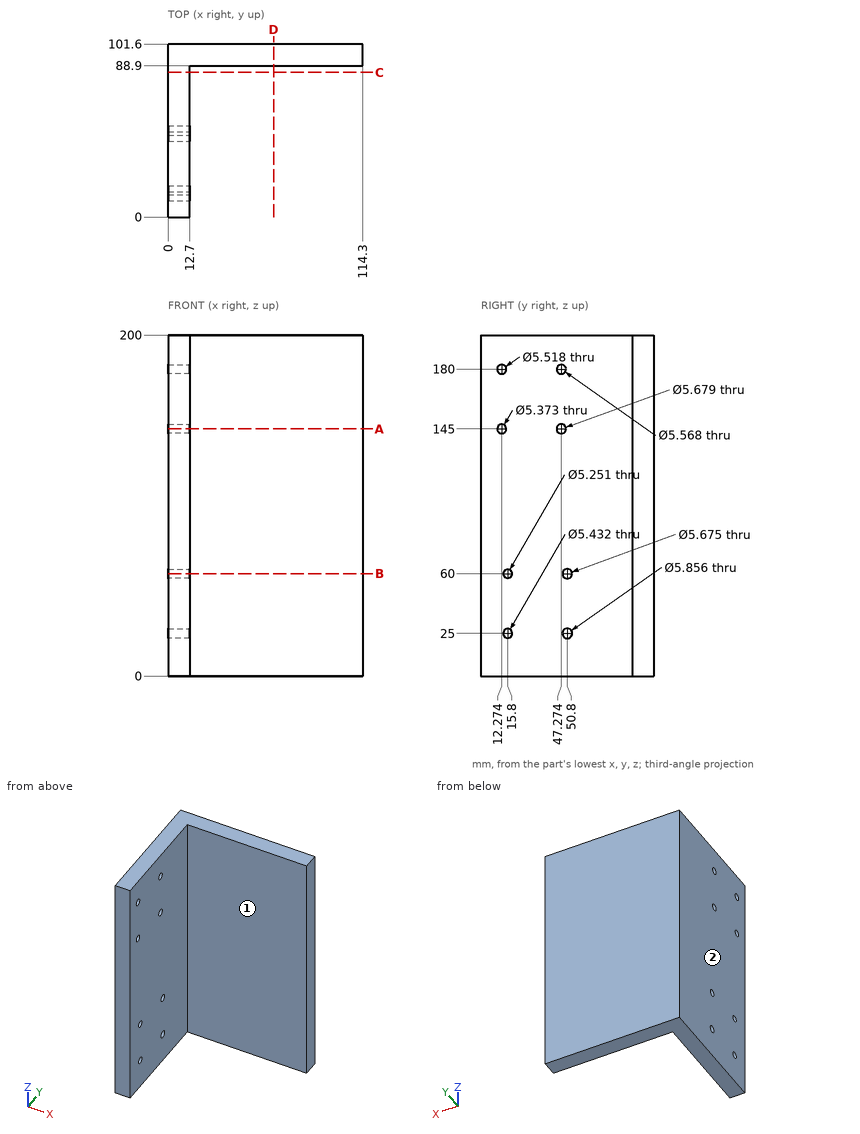
Could you check a few things on this drawing? It's one solid part, dimensions in mm from its lowest x, y, z. A direction names the side the tool comes from. Round coordinates to 2 decimals unless told otherwise and drop trailing zeros. Loops run counter-clockwise (first coordinate to the right, second up) from the corner with the lowest first, then second, coordinate; pieces in that order, holes last. Notation, with made-up numbers: (43, 50.25) -> (47, 50.25) arc R35 cw to (47, 83.25) -> close; hole circle Ø8 at (-14, 56). An arc over 180 degrees is marked (long way). One line per item, written item: value. Start each with the question number.
1. For pin 1 (7 mm diameter, centred on y = 15.8, z = 60, fed in from +X); pin 2 (4.5 mm diameter, centred on y = 50.8, z = 60, fed in from -X); pin 3 (8 mm diameter, centred on x = 56, z = 123.5, fed in from -Y); pin 4 (12 mm diameter, centred on x = 18.5, z = 115, fed in from -Y), each with a flat end and sliding along its axis, tell me the tip position at first contact or that it passes through.
2. If we section it at C-C, the plane y = 85: Write out the boundary of the cut face in (x, z), then the cut area to 3 significant figures.
3. For the marked faces 1 and 2, which set-ups out of +Z, -Z, +X, -X, +Y, -Y let a thin tool reach every point of the face, with its end or its side?
4. If we section it at A-A, the plane z = 145: Write out the boundary of the cut face in (x, y) (1 decimal).
5. If I drill on probe 1 along Y at (x, z) = (3.25, 60) (1 decimal); probe 2 along Y at (x, z) = (3, 180) (1 decimal); probe 3 along X at (y, z) = (62.5, 20), over which ranges is the centre line in solid material (lowest first)?
6. If we section it at B-B, the plane z = 60: Write out the boundary of the cut face in (x, y) (1 decimal), then the cut area to 3 significant figures.
7. If we section it at D-D, the plane x = 62: Write out the boundary of the cut face in (y, z).
Calculated:
1. pin 1: stops at x = 12.7
1. pin 2: passes through
1. pin 3: stops at y = 88.9
1. pin 4: stops at y = 0
2. outline: (0, 0) -> (12.7, 0) -> (12.7, 200) -> (0, 200) -> close
2. area: 2,540 mm²
3. face 1: +Z, -Z, +X, -Y
3. face 2: +Z, -Z, -X, +Y, -Y
4. outline: (0, 0) -> (12.7, 0) -> (12.7, 9.6) -> (0, 9.6) -> close; (0, 15) -> (12.7, 15) -> (12.7, 44.4) -> (0, 44.4) -> close; (0, 50.1) -> (12.7, 50.1) -> (12.7, 88.9) -> (114.3, 88.9) -> (114.3, 101.6) -> (0, 101.6) -> close
5. probe 1: y = 0 to 13.2, 18.4 to 48, 53.6 to 101.6
5. probe 2: y = 0 to 9.5, 15 to 44.5, 50.1 to 101.6
5. probe 3: x = 0 to 12.7
6. outline: (0, 0) -> (12.7, 0) -> (12.7, 13.2) -> (0, 13.2) -> close; (0, 18.4) -> (12.7, 18.4) -> (12.7, 48) -> (0, 48) -> close; (0, 53.6) -> (12.7, 53.6) -> (12.7, 88.9) -> (114.3, 88.9) -> (114.3, 101.6) -> (0, 101.6) -> close
6. area: 2,440 mm²
7. outline: (88.9, 0) -> (101.6, 0) -> (101.6, 200) -> (88.9, 200) -> close
